Autodesk Inventor part; units mm, degrees
ref_plane "YZ Plane" through (0, 0, 0) normal (1, 0, 0) x (0, 1, 0)
ref_plane "XZ Plane" through (0, 0, 0) normal (0, 1, 0) x (-1, 0, 0)
ref_plane "XY Plane" through (0, 0, 0) normal (0, 0, 1) x (1, 0, 0)
sketch "Sketch1" plane through (0, 0, 0) normal (0, 0, 1) x (1, 0, 0)
  line L0 (-15.5, 15.5) -> (15.5, 15.5) construction
  line L1 (15.5, 15.5) -> (15.5, -15.5) construction
  line L2 (15.5, -15.5) -> (-15.5, -15.5) construction
  line L3 (-15.5, -15.5) -> (-15.5, 15.5) construction
  line L4 (-15.5, 15.5) -> (15.5, -15.5) construction
  line L5 (15.5, 15.5) -> (-15.5, -15.5) construction
  circle A0 centre (-15.5, 15.5) radius 2
  circle A1 centre (15.5, 15.5) radius 2
  circle A2 centre (-15.5, -15.5) radius 2
  circle A3 centre (15.5, -15.5) radius 2
  line L6 (-21.25, 21.25) -> (21.25, 21.25)
  line L7 (21.25, 21.25) -> (21.25, -21.25)
  line L8 (21.25, -21.25) -> (-21.25, -21.25)
  line L9 (-21.25, -21.25) -> (-21.25, 21.25)
  line L10 (-21.25, 21.25) -> (21.25, -21.25) construction
  line L11 (21.25, 21.25) -> (-21.25, -21.25) construction
  circle A4 centre (0, 0) radius 15.5
  line L12 (25, -25) -> (-25, -25)
  line L13 (-25, -25) -> (-25, 25)
  line L14 (-25, 25) -> (25, 25)
  line L15 (25, 25) -> (25, -25)
  line L16 (25, -25) -> (-25, 25) construction
  line L17 (-25, -25) -> (25, 25) construction
  dimension "d0" = 31
  dimension "d1" = 31
  dimension "d2" = 4
  dimension "d5" = 31
  dimension "d8" = 31
  dimension "d11" = 42.5
  dimension "d12" = 42.5
  dimension "d13" = 50
  dimension "d14" = 50
extrude "Extrusion1" add sketch "Sketch1" along normal blind 2 contours L6 L7 L8 L9 | L12 L13 L14 L15
extrude "Extrusion2" add sketch "Sketch1" against normal blind 10 contours L12 L13 L14 L15
sketch "Sketch2" plane through (-25, -25, 2) normal (-1, 0, 0) x (0, 0, 1)
  line L0 (0, 0) -> (0, 50) construction
  line L1 (0, 0) -> (-2, 0) construction
  line L2 (-12, 0) -> (0, 0) construction
  line L3 (-2, 40.5) -> (-2, 9.5) construction
  line L4 (-2, 0) -> (-2, 25) construction
  line L5 (-2, 25) -> (-3.5, 25) construction
  line L6 (-5, 37.5) -> (-2, 37.5)
  line L7 (-2, 37.5) -> (-2, 12.5)
  line L8 (-2, 12.5) -> (-5, 12.5)
  line L9 (-5, 12.5) -> (-5, 37.5)
  line L10 (-5, 37.5) -> (-2, 12.5) construction
  line L11 (-2, 37.5) -> (-5, 12.5) construction
  line L12 (-7, 39.5) -> (0, 39.5)
  line L13 (0, 39.5) -> (0, 10.5)
  line L14 (0, 10.5) -> (-7, 10.5)
  line L15 (-7, 10.5) -> (-7, 39.5)
  dimension "d19" = 2
  dimension "d20" = 25
  dimension "d21" = 90
  dimension "d22" = 1.5
  dimension "d23" = 90
  dimension "d24" = 3
  dimension "d25" = 25
  dimension "d26" = 2
  dimension "d37" = 2
extrude "Extrusion3" add sketch "Sketch2" along normal blind 15
sketch "Sketch3" plane through (-25, -14.5, -5) normal (0, 0, -1) x (-1, 0, 0)
  line L0 (0, 0) -> (7.5, 0) construction
  line L1 (0, 0) -> (15, 0) construction
  line L2 (7.5, 14.5) -> (7.5, 21.25) construction
  line L3 (7.5, 21.25) -> (7.5, 7.75) construction
  circle A0 centre (7.5, 21.25) radius 2
  circle A1 centre (7.5, 7.75) radius 2
  line L4 (7.5, 0) -> (7.5, 7.75) construction
  line L5 (7.5, 21.25) -> (7.5, 29) construction
  line L6 (0, 29) -> (15, 29) construction
  point P0 (-25, 14.5)
  dimension "d30" = 4
  dimension "d31" = 4
  dimension "d38" = 13.5
extrude "Extrusion4" cut sketch "Sketch3" against normal blind 15
pattern_circular "Circular Pattern1" count 4 over 360 about axis through (0, 0, -10) along (0, 0, 1) of "Extrusion3", "Extrusion4"
fillet "Fillet2" radius 5 12 edges at (25, 14.5, -1.5) (25, 25, -4) (14.5, 25, -1.5) (25, -14.5, -1.5) (14.5, -25, -1.5) (25, -25, -4) (-14.5, -25, -1.5) (-25, -25, -4) (-25, -14.5, -1.5) (-25, 14.5, -1.5) (-25, 25, -4) (-14.5, 25, -1.5)
properties part number "CSB_Motor_Mount_v1"
Work out the finished part from the listing and answer in its coordinate system (mm). A direction names the side the tool comes from. Give positions to 0.01 mm unless a question says otherwise; leave off trailing zeros. Loops run counter-clockwise (first coordinate to the right, second up) from the corner with the lowest first, then second, coordinate; pieces in that order, holes last. Notation, with made-up numbers: (87.25, 9.25) -> (98.25, 9.25) arc R15 ccw to (98.25, 22.25) -> close; hole circle Ø2 at (-3.5, 47.5). An arc over 180 degrees is marked (long way). Write item = value, one per line. Start each with the question number.
(1) Find section D-D on y = 3.5. Give the vertices of the cut face in (x, z), and give its area (3 significant figures).
(2) Which of the six approach directions +Z, -Z, +X, -X, +Y, -Y give full straight-line access (tool end or side, diameter ignored) to faces 4 (the flat face through (32, 0, 0)), 5 (the flat face through (32, 0, -5)), 6 (the flat face through (9, -14, 0))?
(3) Find the intervals of material crossed by probe 1 along X at (y, z) = (-32.5, 1.65); probe 2 along Y at (x, z) = (6.5, -5.5), in increasing order. Write a range as from..to.
(4) Find section B-B on x = 0. Give the vertices of the cut face in (y, z), and give its area (3 significant figures).
(5) Find section A-A on x = -32.5. Give the vertices of the cut face in (y, z), and give its area (3 significant figures).
(6) Given pin 1 Ø1.5 at (x, z) = (-31.5, -4.5) entering from -Y; pin 2 Ø2 at (y, z) = (35.5, 0) entering from +X; pin 3 Ø1.5 at (y, z) = (5.5, -1.5) entering from +X, each flat-ended and moving along its own axis, determine where each tip first touches the part or whether it passes through.
(7) The mould has two halves that part along X. Classify faces 1 (the cylindrical face through (-24, 23, -4)), 2 (the flat face through (-32, 0, -3)), 3 (the cylindrical face through (-34.408, -6.149, 0.986)): +X half, -X half, draft (parallel to the pull), parting line (faces both ways), or undercut.
(8) Find section C-C on z = -6.5. Give the vertices of the cut face in (x, y).
From the geometry:
q1.outline = (-40, -5) -> (-25, -5) -> (-25, -10) -> (-21.25, -10) -> (-21.25, 0) -> (-15.1, 0) -> (-15.1, 2) -> (-40, 2) -> (-40, 0) -> (-25, 0) -> (-25, -3) -> (-40, -3) -> close; (15.1, 0) -> (21.25, 0) -> (21.25, -10) -> (25, -10) -> (25, -5) -> (40, -5) -> (40, -3) -> (25, -3) -> (25, 0) -> (40, 0) -> (40, 2) -> (15.1, 2) -> close
q1.area = 235 mm^2
q2.face_4 = +X
q2.face_5 = -Z, +X, +Y, -Y
q2.face_6 = -Z
q3.probe_1 = -14.5..-8.75, -4.75..4.75, 8.75..14.5
q3.probe_2 = -25..-21.25, 21.25..25
q4.outline = (-40, -5) -> (-25, -5) -> (-25, -10) -> (-21.25, -10) -> (-21.25, 0) -> (-15.5, 0) -> (-15.5, 2) -> (-40, 2) -> (-40, 0) -> (-25, 0) -> (-25, -3) -> (-40, -3) -> close; (15.5, 0) -> (21.25, 0) -> (21.25, -10) -> (25, -10) -> (25, -5) -> (40, -5) -> (40, -3) -> (25, -3) -> (25, 0) -> (40, 0) -> (40, 2) -> (15.5, 2) -> close
q4.area = 233 mm^2
q5.outline = (-14.5, -5) -> (-8.75, -5) -> (-8.75, -3) -> (-12.5, -3) -> (-12.5, 0) -> (-8.75, 0) -> (-8.75, 2) -> (-14.5, 2) -> close; (-4.75, -5) -> (4.75, -5) -> (4.75, -3) -> (-4.75, -3) -> close; (-4.75, 0) -> (4.75, 0) -> (4.75, 2) -> (-4.75, 2) -> close; (8.75, -5) -> (14.5, -5) -> (14.5, 2) -> (8.75, 2) -> (8.75, 0) -> (12.5, 0) -> (12.5, -3) -> (8.75, -3) -> close
q5.area = 96.0 mm^2
q6.pin_1 = -14.5
q6.pin_2 = 14.5
q6.pin_3 = 25
q7.face_1 = -X half
q7.face_2 = draft
q7.face_3 = undercut
q8.outline = (-25, -20) arc R5 ccw to (-20, -25) -> (20, -25) arc R5 ccw to (25, -20) -> (25, 20) arc R5 ccw to (20, 25) -> (-20, 25) arc R5 ccw to (-25, 20) -> close; hole (-21.25, -21.25) -> (21.25, -21.25) -> (21.25, 21.25) -> (-21.25, 21.25) -> close
